```python
from build123d import *

# Parameters (mm, degrees)
SKETCH_1_W          = 20
SKETCH_1_H          = 20
EXTRUDE_1_DEPTH     = 5
EXTRUDE_2_DEPTH     = 15
EXTRUDE_3_DEPTH     = 15
EXTRUDE_4_DEPTH     = 15
FILLET_1_R          = 1
SKETCH_5_W          = 10
SKETCH_5_H          = 10
CUT_EXTRUDE_1_DEPTH = 1
CUT_EXTRUDE_2_REACH = 40.406
SKETCH_6_R          = 2
CUT_EXTRUDE_3_REACH = 45.875
SKETCH_7_R          = 2
CUT_EXTRUDE_4_REACH = 45.875
SKETCH_8_R          = 2


with BuildPart() as part:
    # 草图1 → 凸台-拉伸1 (new body)
    with BuildSketch(Plane(origin=(0, 0, 0), x_dir=(1, 0, 0), z_dir=(0, 1, 0))):
        Rectangle(SKETCH_1_W, SKETCH_1_H)
    extrude(amount=EXTRUDE_1_DEPTH)

    # 草图2 → 凸台-拉伸2 (add)
    with BuildSketch(Plane.XY.offset(10)):
        Polygon((-3, 5), (3, 5), (5, 1.5), (3, 1.5), (3, 0), (-3, 0), (-3, 1.5), (-5, 1.5), align=None)
    extrude(amount=EXTRUDE_2_DEPTH)

    # 草图3 → 凸台-拉伸3 (add)
    with BuildSketch(Plane.ZY.offset(10)):
        Polygon((-3, 5), (3, 5), (5, 1.5), (3, 1.5), (3, 0), (-3, 0), (-3, 1.5), (-5, 1.5), align=None)
    extrude(amount=EXTRUDE_3_DEPTH)

    # 草图4 → 凸台-拉伸4 (add)
    with BuildSketch(Plane(origin=(0, 5, 0), x_dir=(1, 0, 0), z_dir=(0, 1, 0))):
        Polygon((-3, 10), (-3, 8.5), (-5, 8.5), (-3, 5), (3, 5), (5, 8.5), (3, 8.5), (3, 10), align=None)
        Polygon((8.5, -5), (5, -3), (5, 3), (8.5, 5), (8.5, 3), (10, 3), (10, -3), (8.5, -3), align=None)
    extrude(amount=EXTRUDE_4_DEPTH)

    # 圆角1
    fillet_1_edges = [part.edges().sort_by_distance(p)[0] for p in [
        (10, 2.5, 10),
        (-10, 2.5, 10),
        (-10, 2.5, -10),
        (10, 2.5, -10),
    ]]
    fillet(fillet_1_edges, radius=FILLET_1_R)

    # 草图5 → 切除-拉伸1 (cut)
    with BuildSketch(Plane(origin=(0, 5, 0), x_dir=(1, 0, 0), z_dir=(0, 1, 0))):
        Rectangle(SKETCH_5_W, SKETCH_5_H)
    extrude(amount=-CUT_EXTRUDE_1_DEPTH, mode=Mode.SUBTRACT)

    # 草图6 → 切除-拉伸2 (cut, up to next)
    with BuildSketch(Plane(origin=(0, 5, 0), x_dir=(1, 0, 0), z_dir=(0, 1, 0)), mode=Mode.PRIVATE) as cut_extrude_2_sk1:
        with Locations(Location((0, -19.5, 0), (0, 0, 270))):
            Circle(SKETCH_6_R)
    cut_extrude_2_tool1 = extrude(cut_extrude_2_sk1.sketch, amount=-CUT_EXTRUDE_2_REACH, mode=Mode.PRIVATE) & part.part
    # 草图6 → 切除-拉伸2 (cut, up to next)
    with BuildSketch(Plane(origin=(0, 5, 0), x_dir=(1, 0, 0), z_dir=(0, 1, 0)), mode=Mode.PRIVATE) as cut_extrude_2_sk2:
        with Locations(Location((-19.5, 0, 0), (0, 0, 270))):
            Circle(SKETCH_6_R)
    cut_extrude_2_tool2 = extrude(cut_extrude_2_sk2.sketch, amount=-CUT_EXTRUDE_2_REACH, mode=Mode.PRIVATE) & part.part
    add(cut_extrude_2_tool1.solids().sort_by_distance((0, 5, 19.5))[0], mode=Mode.SUBTRACT)
    add(cut_extrude_2_tool2.solids().sort_by_distance((-19.5, 5, 0))[0], mode=Mode.SUBTRACT)

    # 草图7 → 切除-拉伸3 (cut, up to next)
    with BuildSketch(Plane.ZY.offset(-5), mode=Mode.PRIVATE) as cut_extrude_3_sk1:
        with Locations((0, 14.5)):
            Circle(SKETCH_7_R)
    cut_extrude_3_tool1 = extrude(cut_extrude_3_sk1.sketch, amount=-CUT_EXTRUDE_3_REACH, mode=Mode.PRIVATE) & part.part
    add(cut_extrude_3_tool1.solids().sort_by_distance((5, 14.5, 0))[0], mode=Mode.SUBTRACT)

    # 草图8 → 切除-拉伸4 (cut, up to next)
    with BuildSketch(Plane.XY.offset(-5), mode=Mode.PRIVATE) as cut_extrude_4_sk1:
        with Locations((0, 14.5)):
            Circle(SKETCH_8_R)
    cut_extrude_4_tool1 = extrude(cut_extrude_4_sk1.sketch, amount=-CUT_EXTRUDE_4_REACH, mode=Mode.PRIVATE) & part.part
    add(cut_extrude_4_tool1.solids().sort_by_distance((0, 14.5, -5))[0], mode=Mode.SUBTRACT)


solid = part.part
```
Check sheet for the modelled part. Datum: model origin and axes. Units: mm. A direction names the side the tool comes from. Round coordinates to 2 decimals unless told otherwise and drop trailing zeros. Order: outer loops, then holes, each group sorted by start corner. A loop starts at its lowest first (then second) coordinate and runs counter-clockwise, first axis right, second up. Notation, with made-up numbers: (74.5, 62.5) - (129.5, 62.5) arc R26 ccw to (129.5, 88.5) - close; hole circle Ø5 at (27, 28.25). An arc over 180 degrees is marked (long way). Answer as CSV lines item,"result". Start each with the question number.
1) Section check A-A (y = 14.5). Record the cut outline in (x, z), then the cut area to 3 significant figures.
2) Section check C-C (y = 7.5). Record the cut outline in (x, z).
3) Draft check along Z on faces 1 (the face through (10, 8, 0)), 2 (the face through (4, 12, -8.5)), 3 (the face through (7.465, 16.483, -0.26)). Enter one of: +Z half, -Z half, draft (parallel to the pull), parting line (faces both ways), or undercut.
4) Tool access check on faces 4 (the face through (0, 4, 0)), 5 (the face through (3, 1, 17)), 6 (the face through (3.99, 3.27, 17.4)), 7 (the face through (-3, 1, 17)), 8 (the face through (3, 12, -9)). Record the directions out of +Z, -Z, +X, -X, +Y, -Y that give a thin tool (end or side, any length) a straight path to the whole face; none if there is none.
5) Section check D-D (x = -19.5). Record the cut outline in (y, z), then the cut area to 3 significant figures.
6) Scan lines: probe 1 along Y at (x, z) = (0, -7.2); probe 2 along X at (y, z) = (12, 0.5); probe 3 along Y at (x, z) = (-10.5, -0.5). Record each from-to range of solid material in increasing order.
7) Section check B-B (z = 0). Record the cut outline in (x, y).
8) Depth check by flat-ended pin: pin 1 (3 mm diameter, centred on x = -8.5, z = 2.5, fed in from -Y); pin 2 (1.6 mm diameter, centred on x = 4, z = 17.5, fed in from -Y); pin 3 (6 mm diameter, centred on x = -19.5, z = 2.5, fed in from +Y); pin 4 (10 mm diameter, centred on x = -16.5, y = 4.5, fed in from +Z). Enter the tip coordinate at first touch or a pass-through.
Determined:
1,outline,"(-5, -8.5) - (-3, -8.5) - (-3, -10) - (-2, -10) - (-2, -5) - (-3, -5) - close; (2, -10) - (3, -10) - (3, -8.5) - (5, -8.5) - (3, -5) - (2, -5) - close; (5, -3) - (8.5, -5) - (8.5, -3) - (10, -3) - (10, -2) - (5, -2) - close; (5, 2) - (10, 2) - (10, 3) - (8.5, 3) - (8.5, 5) - (5, 3) - close"
1,area,"34.0 mm^2"
2,outline,"(-5, -8.5) - (-3, -8.5) - (-3, -10) - (3, -10) - (3, -8.5) - (5, -8.5) - (3, -5) - (-3, -5) - close; (5, -3) - (8.5, -5) - (8.5, -3) - (10, -3) - (10, 3) - (8.5, 3) - (8.5, 5) - (5, 3) - close"
3,face 1,"draft"
3,face 2,"-Z half"
3,face 3,"undercut"
4,face 4,"+Y"
4,face 5,"+Z, +X, -Y"
4,face 6,"+Z, +X, +Y"
4,face 7,"+Z, -X, -Y"
4,face 8,"-Z, +X, +Y"
5,outline,"(0, -3) - (1.5, -3) - (1.5, -5) - (5, -3) - (5, -2) - (0, -2) - close; (0, 2) - (5, 2) - (5, 3) - (1.5, 5) - (1.5, 3) - (0, 3) - close"
5,area,"17.0 mm^2"
6,probe 1,"0 to 12.5, 16.5 to 20"
6,probe 2,"5 to 10"
6,probe 3,"0 to 5"
7,outline,"(-25, 0) - (-21.5, 0) - (-21.5, 5) - (-25, 5) - close; (-17.5, 0) - (10, 0) - (10, 12.5) - (5, 12.5) - (5, 4) - (-5, 4) - (-5, 5) - (-17.5, 5) - close; (5, 16.5) - (10, 16.5) - (10, 20) - (5, 20) - close"
8,pin 1,"y = 0"
8,pin 2,"y = 1.5"
8,pin 3,"y = 5"
8,pin 4,"z = 5"
